Can you work these out from the model? Positions are in its coordinate system, mm. A direction names the side the tool comes from. Coordinates: 2 decimals unless noted, no trailing zeros. Write each loop counter-clockwise with the first axis right and the second up, starting at its lowest first coordinate (ties: lowest second). Pieces come first, ordered by that corner, then holes. Notation, with made-up numbers: (52, 33) -> (75, 33) arc R23 ccw to (75, 48) -> close; hole circle Ø10 at (83, -39.75). An arc over 180 degrees is marked (long way). Use one line per item in the form item = value.
Autodesk Inventor part; units mm, degrees
ref_plane "YZ Plane" through (0, 0, 0) normal (1, 0, 0) x (0, 1, 0)
ref_plane "XZ Plane" through (0, 0, 0) normal (0, 1, 0) x (-1, 0, 0)
ref_plane "XY Plane" through (0, 0, 0) normal (0, 0, 1) x (1, 0, 0)
sketch "Sketch1" plane through (0, 0, 0) normal (0, 1, 0) x (-1, 0, 0)
  line L0 (30, -26.5) -> (-30, -26.5)
  line L1 (-30, -26.5) -> (-30, 26.5)
  line L2 (-30, 26.5) -> (30, 26.5)
  line L3 (30, 26.5) -> (30, -26.5)
  line L4 (30, -26.5) -> (-30, 26.5) construction
  line L5 (-30, -26.5) -> (30, 26.5) construction
  line L6 (-3, 21) -> (-25, 21) construction
  line L7 (-25, 21) -> (-25, 10.7) construction
  line L8 (-25, 10.7) -> (-3, 10.7) construction
  line L9 (-3, 10.7) -> (-3, 21) construction
  line L10 (0, 0) -> (30, 0)
  line L11 (0, 0) -> (0, -26.5)
  point P0 (-14, -18.5)
  point P1 (-14, 10.7)
  point P2 (22, 11.5)
  dimension "d0" = 60
  dimension "d1" = 53
  dimension "d2" = 5
  dimension "d3" = 5.5
  dimension "d4" = 22
  dimension "d5" = 10.3
  dimension "d6" = 45
  dimension "d7" = 8
  dimension "d8" = 15
extrude "Extrusion1" add sketch "Sketch1" along normal blind 5 contours L0 L1 L2 L3 L10 L11
hole "Hole1" at (3, 0, 21) at (25, 0, 10.7) direction (0, 1, 0) diameter 2.7 end through all
hole "Hole2" at (14, 0, -18.5) at (-22, 0, 11.5) direction (0, 1, 0) diameter 6.1 end through all
fillet "Fillet1" radius 3 6 edges at (-30, 2.5, 26.5) (30, 2.5, 26.5) (30, 2.5, -26.5) (0, 2.5, -26.5) (0, 2.5, 0) (-30, 2.5, 0)
properties part number "Limit SW Bracket Left" material "ABS Plastic"
Q1. Suppose I cut it at C-C (y = 4.35). Write out the boundary of the cut face in (x, z), then the cut area to 3 significant figures.
Return value:
outline = (-30, 3) arc R3 ccw to (-27, 0) -> (-3, 0) arc R3 cw to (0, -3) -> (0, -23.5) arc R3 ccw to (3, -26.5) -> (27, -26.5) arc R3 ccw to (30, -23.5) -> (30, 23.5) arc R3 ccw to (27, 26.5) -> (-27, 26.5) arc R3 ccw to (-30, 23.5) -> close; hole circle Ø6.1 at (-22, 11.5); hole circle Ø2.7 at (3, 21); hole circle Ø6.1 at (14, -18.5); hole circle Ø2.7 at (25, 10.7)
area = 2,310 mm2
Q2. Will these pins go through, and if not, where does the flat tip stop? pin 1 (1.5 mm diameter, centred on x = -17, y = 2.5, fed in from -Z); pin 2 (1 mm diameter, centred on y = 2.5, z = -21, fed in from -X); pin 3 (2.5 mm diameter, centred on x = 3, z = 21, fed in from +Y).
Return value:
pin_1 = 0
pin_2 = 0
pin_3 = through
Q3. Suppose I cut it at A-A (x = -22). Write out the boundary of the cut face in (y, z).
Return value:
outline = (0, 0) -> (5, 0) -> (5, 8.45) -> (0, 8.45) -> close; (0, 14.55) -> (5, 14.55) -> (5, 26.5) -> (0, 26.5) -> close
Q4. Suppose I cut it at B-B (z = -18.5). Write out the boundary of the cut face in (x, y).
Return value:
outline = (0, 0) -> (10.95, 0) -> (10.95, 5) -> (0, 5) -> close; (17.05, 0) -> (30, 0) -> (30, 5) -> (17.05, 5) -> close
Q5. Suppose I cut it at D-D (z = 10.7). Write out the boundary of the cut face in (x, y), then the cut area to 3 significant figures.
Return value:
outline = (-30, 0) -> (-24.94, 0) -> (-24.94, 5) -> (-30, 5) -> close; (-19.06, 0) -> (23.65, 0) -> (23.65, 5) -> (-19.06, 5) -> close; (26.35, 0) -> (30, 0) -> (30, 5) -> (26.35, 5) -> close
area = 257 mm2
Q6. For faces 4 (the flat face through (0, 2, -13)), 5 (the cylindrical face through (29.1, 2.54, 25.64)), which set-ups out of +Z, -Z, +X, -X, +Y, -Y let a thin tool reach every point of the face, with its end or its side?
Return value:
face_4 = -Z, -X, +Y, -Y
face_5 = +Z, +X, +Y, -Y
Q7. Thinking about a two-plate mould opening in X: for faces 1 (the cylindrical face through (25.517, 2.535, 9.453)), 2 (the flat face through (0, 2, 26.5)), 3 (the cylindrical face through (-29.1, 2.54, 0.86)), which applies, released by +X, released by -X, zero draft, split by the parting line, or undercut?
Return value:
face_1 = undercut
face_2 = zero draft
face_3 = released by -X
Q8. If I drill on line 1 (X direction, y = 1.3, z = 21); line 2 (Z direction, x = 25, y = 3.25); line 3 (Z direction, x = 3, y = 3.9), over which ranges is the centre line in solid material (lowest first)? Write a range as from..to.
Return value:
line_1 = -30..1.65, 4.35..30
line_2 = -26.5..9.35, 12.05..26.5
line_3 = -26.5..19.65, 22.35..26.5
